The listing builds one solid part. Answer for the finished solid, in the listing's coordinates (mm). Coordinates: 2 decimals unless noted, no trailing zeros. Put each result on its own line as item: value.
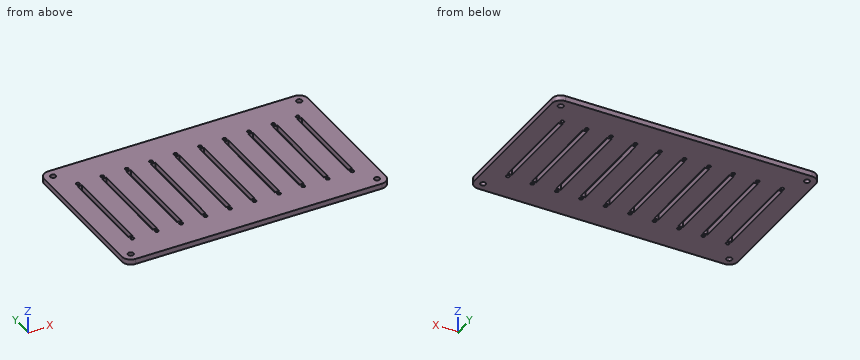
```python
from build123d import *

# Parameters (mm, degrees)
PAD_DEPTH           = 3
SKETCH002_R         = 1
SKETCH002_W         = 2.5
SKETCH002_H         = 52
POCKET_DEPTH        = 3.001
LINEARPATTERN_COUNT = 10
LINEARPATTERN_PITCH = 13.888889
SKETCH003_R         = 1.55
POCKET001_DEPTH     = 3.001


with BuildPart() as part:
    # Sketch → Pad (new body)
    with BuildSketch(Plane.XY):
        with BuildLine():
            Line((-70, 45), (70, 45))
            ThreePointArc((75, 40), (73.535534, 43.535534), (70, 45))
            Line((75, 40), (75, -40))
            ThreePointArc((70, -45), (73.535534, -43.535534), (75, -40))
            Line((70, -45), (-70, -45))
            ThreePointArc((-75, -40), (-73.535534, -43.535534), (-70, -45))
            Line((-75, -40), (-75, 40))
            ThreePointArc((-70, 45), (-73.535534, 43.535534), (-75, 40))
        make_face()
    extrude(amount=PAD_DEPTH)

    # Sketch002 → Pocket (cut, through all)
    with BuildSketch(Plane(origin=(-62.5, 0, 0), x_dir=(1, 0, 0), z_dir=(0, 0, 1))):
        with Locations((0, 28)):
            Circle(SKETCH002_R)
        with Locations((0, -28)):
            Circle(SKETCH002_R)
        Rectangle(SKETCH002_W, SKETCH002_H)
    pocket = extrude(amount=POCKET_DEPTH, mode=Mode.SUBTRACT)

    # LinearPattern: Pocket ×10
    with Locations(*[(i * LINEARPATTERN_PITCH, 0, 0) for i in range(1, LINEARPATTERN_COUNT)]):
        add(pocket, mode=Mode.SUBTRACT)

    # Sketch003 → Pocket001 (cut, through all)
    with BuildSketch(Plane.XY):
        with Locations((-70, 40)):
            Circle(SKETCH003_R)
        with Locations((-70, -40)):
            Circle(SKETCH003_R)
        with Locations((70, 40)):
            Circle(SKETCH003_R)
        with Locations((70, -40)):
            Circle(SKETCH003_R)
    extrude(amount=POCKET001_DEPTH, mode=Mode.SUBTRACT)


solid = part.part
```
1) The part is cut by section A-A (y = -9). State how many separate pieces and enclosed holes the cut face has, and give its area (3 significant figures).
Found:
separate pieces: 11
enclosed holes: 0
area: 375 mm^2
2) Straight lines are drawn through the part: L1, parallel to X at y = 40, z = 2.1; L2, parallel to Y at x = -62.5, z = 1.9. For each, find the intervals that lie inside material, in ascending order. Write a range as [from, to].
Found:
L1: x = [-75, -71.55], [-68.45, 68.45], [71.55, 75]
L2: y = [-45, -29], [-27, -26], [26, 27], [29, 45]
3) This flat-tipped pin is pushed along its axis until it touches: pin 1 (2.5 mm diameter, centred on x = -62.5, y = 28, fed in from -Z). Where does it stop, or does it pass through?
Found:
pin 1: stops at z = 0
